CAD build for the part. Positions are in the model's coordinates, mm. Coordinates: 2 decimals unless noted, no trailing zeros. Loops run counter-clockwise (first coordinate to the right, second up) from the corner with the lowest first, then second, coordinate; pieces in that order, holes last. Notation, with made-up numbers: (-29.5, 4) -> (0.5, 4) arc R35 cw to (0.5, 42) -> close; hole circle Ø2 at (4, -26). An arc over 180 degrees is marked (long way). Answer as a JSON object with one key per item and string values. Group by question number.
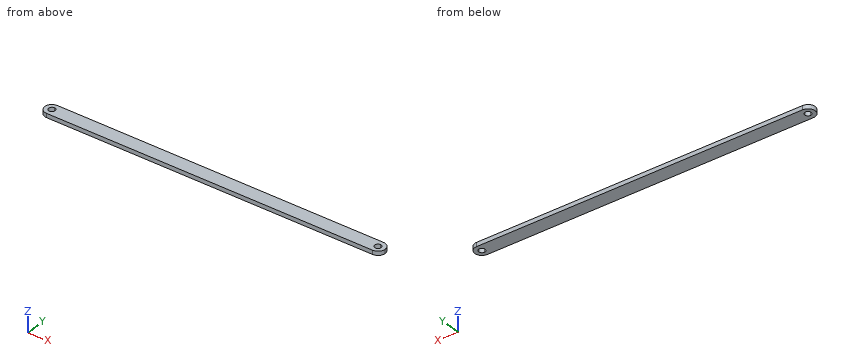
from build123d import *

# Parameters (mm, degrees)
BOSS_EXTRUDE1_DEPTH = 2.54


with BuildPart() as part:
    # Sketch1 → Boss-Extrude1 (new body)
    with BuildSketch(Plane.XY):
        with BuildLine():
            Line((101.6, 4.445), (-101.6, 4.445))
            ThreePointArc((-101.6, 4.445), (-98.456910358, 3.143089642), (-97.155, 0))
            ThreePointArc((-97.155, 0), (-98.456910358, -3.143089642), (-101.6, -4.445))
            Line((-101.6, -4.445), (101.6, -4.445))
            ThreePointArc((101.6, -4.445), (97.155, 0), (101.6, 4.445))
        make_face()
        with BuildLine():
            ThreePointArc((-97.155, 0), (-98.456910358, 3.143089642), (-101.6, 4.445))
            Line((-101.6, 4.445), (-101.6, 1.9939))
            ThreePointArc((-101.6, 1.9939), (-100.190099789, 1.409900211), (-99.6061, 0))
            ThreePointArc((-99.6061, 0), (-100.190099789, -1.409900211), (-101.6, -1.9939))
            Line((-101.6, -1.9939), (-101.6, -4.445))
            ThreePointArc((-101.6, -4.445), (-98.456910358, -3.143089642), (-97.155, 0))
        make_face()
        with BuildLine():
            Line((-101.6, 1.9939), (-101.6, 4.445))
            ThreePointArc((-101.6, 4.445), (-106.045, 0), (-101.6, -4.445))
            Line((-101.6, -4.445), (-101.6, -1.9939))
            ThreePointArc((-101.6, -1.9939), (-103.5939, 0), (-101.6, 1.9939))
        make_face()
        with BuildLine():
            ThreePointArc((106.045, 0), (104.743089642, 3.143089642), (101.6, 4.445))
            Line((101.6, 4.445), (101.6, 1.9939))
            ThreePointArc((101.6, 1.9939), (103.009900211, 1.409900211), (103.5939, 0))
            ThreePointArc((103.5939, 0), (103.009900211, -1.409900211), (101.6, -1.9939))
            Line((101.6, -1.9939), (101.6, -4.445))
            ThreePointArc((101.6, -4.445), (104.743089642, -3.143089642), (106.045, 0))
        make_face()
        with BuildLine():
            Line((101.6, 1.9939), (101.6, 4.445))
            ThreePointArc((101.6, 4.445), (97.155, 0), (101.6, -4.445))
            Line((101.6, -4.445), (101.6, -1.9939))
            ThreePointArc((101.6, -1.9939), (99.6061, 0), (101.6, 1.9939))
        make_face()
    extrude(amount=BOSS_EXTRUDE1_DEPTH)


solid = part.part
Item 1: Drill centre lines: L1, parallel to X at y = 0.25, z = 0.8; L2, parallel to X at y = 1.25, z = 0.6; L3, parallel to X at y = -2.5, z = 1.8. Where is each one in solid material? Low to high.
Item 2: Band-saw the part on A-A, the plane z = 1.55. List the corners of the cut face in (x, y) (3 decimals).
Item 3: Flat gauge pin, fed straight in: P1, Ø1, axis at y = 1, z = 0.5, coming from the +X side. Where does the tip first touch, or does it go through?
Reply:
{
 "1": {"L1": "-106.04 to -103.58, -99.62 to 99.62, 103.58 to 106.04", "L2": "-105.87 to -103.15, -100.05 to 100.05, 103.15 to 105.87", "L3": "-105.28 to 105.28"},
 "2": {"outline": "(-101.6, -4.445) -> (101.6, -4.445) arc R4.445 ccw to (101.6, 4.445) -> (-101.6, 4.445) arc R4.445 ccw to start; hole circle Ø3.988 at (-101.6, 0); hole circle Ø3.988 at (101.6, 0)"},
 "3": {"P1": "x = 106.02"}
}
